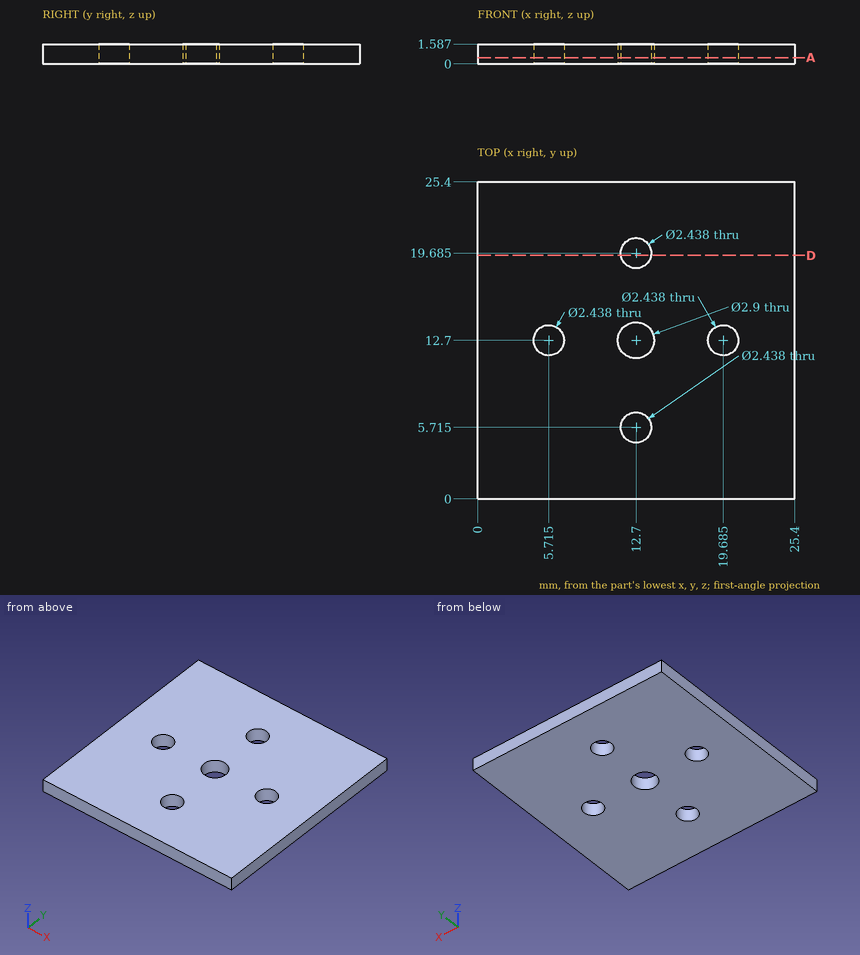
For this review, use the dimensioned drawing (mm, ordinates from the lowest corner) and the shaded views. Coordinates: 2 decimals unless noted, no trailing zeros. Loops run counter-clockwise (first coordinate to the right, second up) from the corner with the lowest first, then second, coordinate; pieces in that order, holes last.
1. Add section D-D, the plane y = 19.5. Give the boundary of the cut face in (x, z) (1 decimal).
2. For line 1 (X direction, y = 13, z = 1); line 2 (X direction, y = 19, z = 0.85); line 3 (Y direction, x = 5.5, z = 0.15), list the stretches that pass through material, from the lowest coordinate up.
3. Add section A-A, the plane z = 0.5. Count the separate pieces of the cut face and the enclosed holes in it, then the cut area to 3 significant figures.
Result:
1. outline: (0, 0) - (11.5, 0) - (11.5, 1.6) - (0, 1.6) - close; (13.9, 0) - (25.4, 0) - (25.4, 1.6) - (13.9, 1.6) - close
2. line 1: x = 0 to 4.53, 6.9 to 11.28, 14.12 to 18.5, 20.87 to 25.4
2. line 2: x = 0 to 11.69, 13.71 to 25.4
2. line 3: y = 0 to 11.5, 13.9 to 25.4
3. separate pieces: 1
3. enclosed holes: 5
3. area: 620 mm2
